```python
from build123d import *

# Parameters (mm, degrees)
SKETCH_1_R          = 6.75
SKETCH_1_R_2        = 2.6
EXTRUDE_1_DEPTH     = 3
SKETCH_2_R          = 1.6
CUT_EXTRUDE_1_DEPTH = 10
SKETCH_3_W          = 59.357674729
SKETCH_3_H          = 17.816533783
CUT_EXTRUDE_2_DEPTH = 10
FILLET_1_R          = 2


with BuildPart() as part:
    # 草图1 → 凸台-拉伸1 (new body)
    with BuildSketch(Plane.XY):
        with BuildLine():
            Line((2, 0), (48, 0))
            ThreePointArc((48, 0), (49.414213562, -0.585786438), (50, -2))
            Line((50, -2), (50, -40))
            ThreePointArc((50, -40), (49.414213562, -41.414213562), (48, -42))
            Line((48, -42), (2, -42))
            ThreePointArc((2, -42), (0.585786438, -41.414213562), (0, -40))
            Line((0, -40), (0, -2))
            ThreePointArc((0, -2), (0.585786438, -0.585786438), (2, 0))
        make_face()
        with Locations((25, -21)):
            Circle(SKETCH_1_R, mode=Mode.SUBTRACT)
        with Locations((43, -21)):
            Circle(SKETCH_1_R_2, mode=Mode.SUBTRACT)
        with Locations(Location((7, -21, 0), (0, 0, 180))):
            Circle(SKETCH_1_R_2, mode=Mode.SUBTRACT)
    extrude(amount=EXTRUDE_1_DEPTH)

    # 草图2 → 切除-拉伸1 (cut)
    with BuildSketch(Plane(origin=(0, 0, 0), x_dir=(-1, 0, 0), z_dir=(0, 0, -1))):
        with Locations((-19, -38)):
            Circle(SKETCH_2_R)
        with Locations((-31, -38)):
            Circle(SKETCH_2_R)
    extrude(amount=-CUT_EXTRUDE_1_DEPTH, mode=Mode.SUBTRACT)

    # 草图3 → 切除-拉伸2 (cut)
    with BuildSketch(Plane.XY.offset(3)):
        with Locations((23.80492675, 1.408266891)):
            Rectangle(SKETCH_3_W, SKETCH_3_H)
    extrude(amount=-CUT_EXTRUDE_2_DEPTH, mode=Mode.SUBTRACT)

    # 圆角1
    fillet_1_edges = [part.edges().sort_by_distance(p)[0] for p in [
        (50, -7.5, 1.5),
        (0, -7.5, 1.5),
    ]]
    fillet(fillet_1_edges, radius=FILLET_1_R)


solid = part.part
```
Source: CAD feature listing. Evaluate the final solid. Frame: model axes, mm. Coordinates: 2 decimals unless noted, no trailing zeros. Order: outer loops, then holes, each group sorted by start corner. A loop starts at its lowest first (then second) coordinate and runs counter-clockwise, first axis right, second up. Notation, with made-up numbers: (54, 60) - (81, 60) arc R23 ccw to (81, 70) - close; hole circle Ø5 at (26, 11.5). An arc over 180 degrees is marked (long way). One line per item, written item: value.
1) Contact query for a flat-ended pin moving along its axis: pin 1 (3 mm diameter, centred on x = 32, y = -30.5, fed in from -Z). Output: stop coordinate, or through.
Computed values:
pin 1: stops at z = 0
2) Ray query, line 1 (Y direction, x = 31, z = 2.2); line 2 (X direction, y = -20, z = 1.7); line 3 (Y direction, x = 30, z = 0.9). Return the intervals inside material, ascending. Write a range as [from, to].
Computed values:
line 1: y = [-42, -39.6], [-36.4, -24.09], [-17.91, -7.5]
line 2: x = [0, 4.6], [9.4, 18.32], [31.68, 40.6], [45.4, 50]
line 3: y = [-42, -39.25], [-36.75, -25.53], [-16.47, -7.5]
3) Cut plane D-D on z = 1.05. Output: boundary loops of the cut face in (x, y), plus the area to 3 significant figures.
Computed values:
outline: (0, -40) arc R2 ccw to (2, -42) - (48, -42) arc R2 ccw to (50, -40) - (50, -9.5) arc R2 ccw to (48, -7.5) - (2, -7.5) arc R2 ccw to (0, -9.5) - close; hole circle Ø5.2 at (7, -21); hole circle Ø3.2 at (19, -38); hole circle Ø13.5 at (25, -21); hole circle Ø3.2 at (31, -38); hole circle Ø5.2 at (43, -21)
area: 1,520 mm^2
4) Cut plane C-C on y = -38. Output: boundary loops of the cut face in (x, z).
Computed values:
outline: (0, 0) - (17.4, 0) - (17.4, 3) - (0, 3) - close; (20.6, 0) - (29.4, 0) - (29.4, 3) - (20.6, 3) - close; (32.6, 0) - (50, 0) - (50, 3) - (32.6, 3) - close
5) Cut plane B-B on y = -21. Output: boundary loops of the cut face in (x, z).
Computed values:
outline: (0, 0) - (4.4, 0) - (4.4, 3) - (0, 3) - close; (9.6, 0) - (18.25, 0) - (18.25, 3) - (9.6, 3) - close; (31.75, 0) - (40.4, 0) - (40.4, 3) - (31.75, 3) - close; (45.6, 0) - (50, 0) - (50, 3) - (45.6, 3) - close
6) Cut plane A-A on x = 43. Output: boundary loops of the cut face in (y, z).
Computed values:
outline: (-42, 0) - (-23.6, 0) - (-23.6, 3) - (-42, 3) - close; (-18.4, 0) - (-7.5, 0) - (-7.5, 3) - (-18.4, 3) - close
7) Mould query, pull axis Y, two halves, no side actions, for faces 1 (the face through (25, -28, 0)), 2 (the face through (7.338, -23.578, 1.479)), 3 (the face through (0.57, -8.1, 1.52)). Classes: released by +Y, released by -Y, zero draft, split by the parting line, or undercut.
Computed values:
face 1: zero draft
face 2: undercut
face 3: released by +Y
